For this review, take the finished solid that the model builds, in its own axes (mm). Face numbers are marked on the shaded views. Give positions to 0.01 mm unless a question says otherwise; leave off trailing zeros. Order: outer loops, then holes, each group sorted by start corner. A loop starts at its lowest first (then second) coordinate and runs counter-clockwise, first axis right, second up. Notation, with made-up numbers: (2.25, 41) -> (61.25, 41) arc R29 ccw to (61.25, 61) -> close; hole circle Ø1 at (-26, -7.5). An arc over 180 degrees is marked (long way). Use CSV: the item, a comma, the result in double quotes. Start each with the question number.
Autodesk Inventor part; units mm, degrees
ref_plane "YZ Plane" through (0, 0, 0) normal (1, 0, 0) x (0, 1, 0)
ref_plane "XZ Plane" through (0, 0, 0) normal (0, 1, 0) x (-1, 0, 0)
ref_plane "XY Plane" through (0, 0, 0) normal (0, 0, 1) x (1, 0, 0)
sketch "Szkic1" plane through (0, 0, 0) normal (0, 0, 1) x (1, 0, 0)
  line L0 (-10, 14) -> (0, 14)
  line L1 (0, 14) -> (0, 0)
  line L2 (0, 0) -> (-10, 0)
  line L3 (-10, 0) -> (-10, 14)
  point P0 (-5, 9)
  dimension "d0" = 10
  dimension "d5" = 5
  dimension "d6" = 5
  dimension "d7" = 9
extrude "Wyciągnięcie proste1" add sketch "Szkic1" along normal mid plane 1
fillet "Zaokrąglenie1" radius 5 2 edges at (0, 14, 0) (-10, 14, 0)
hole "Otwór1" at (-5, 9, 0) direction (0, 0, 1) diameter 3 end through all both
properties part number "podporka"
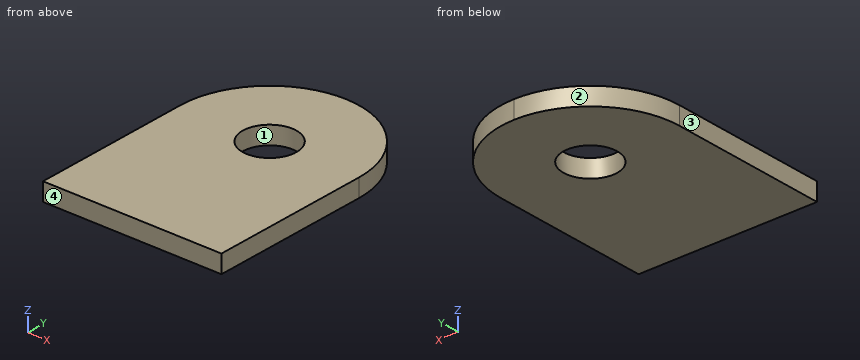
1. Consider section D-D (x = -4.75). State the section outline as (y, z) points, plus the area to 3 significant figures.
2. Consider section B-B (x = -6). State the section outline as (y, z) points, plus the area to 3 significant figures.
3. To check wall thickness, follow L1, parallel to X at y = 9, z = -0.2; L2, parallel to Y at x = -5, z = 0.15; L3, parallel to Y at x = -5.5, z = -0.15. State the ranges of each line that lie inside material, in increasing order. Write a range as [from, to].
4. Consider section C-C (y = 11.25). State the section outline as (x, z) points, plus the area to 3 significant figures.
5. Draft analysis for pull direction Y (two halves, no side actions). For the marked faces 1, 2, 3 and 4, state which applies: +Y half, -Y half, draft (parallel to the pull), parting line (faces both ways), or undercut.
Answer list:
1,outline,"(0, -0.5) -> (7.52, -0.5) -> (7.52, 0.5) -> (0, 0.5) -> close; (10.48, -0.5) -> (13.99, -0.5) -> (13.99, 0.5) -> (10.48, 0.5) -> close"
1,area,"11.0 mm2"
2,outline,"(0, -0.5) -> (7.88, -0.5) -> (7.88, 0.5) -> (0, 0.5) -> close; (10.12, -0.5) -> (13.9, -0.5) -> (13.9, 0.5) -> (10.12, 0.5) -> close"
2,area,"11.7 mm2"
3,L1,"[-10, -6.5], [-3.5, 0]"
3,L2,"[0, 7.5], [10.5, 14]"
3,L3,"[0, 7.59], [10.41, 13.97]"
4,outline,"(-9.47, -0.5) -> (-0.53, -0.5) -> (-0.53, 0.5) -> (-9.47, 0.5) -> close"
4,area,"8.93 mm2"
5,face 1,"undercut"
5,face 2,"+Y half"
5,face 3,"draft"
5,face 4,"-Y half"
